Work out the finished part from the listing and answer in its coordinate system (mm). Face numbers are marked on the shaded views. Coordinates: 2 decimals unless noted, no trailing zeros. Order: outer loops, then holes, each group sorted by start corner. A loop starts at its lowest first (then second) coordinate and runs counter-clockwise, first axis right, second up. Notation, with made-up numbers: M -4,8.5 L 5,8.5 A15 cw 5,31.5 Z; hole C 23,85 d11. An arc over 180 degrees is marked long. Use a Markdown table: item, result.
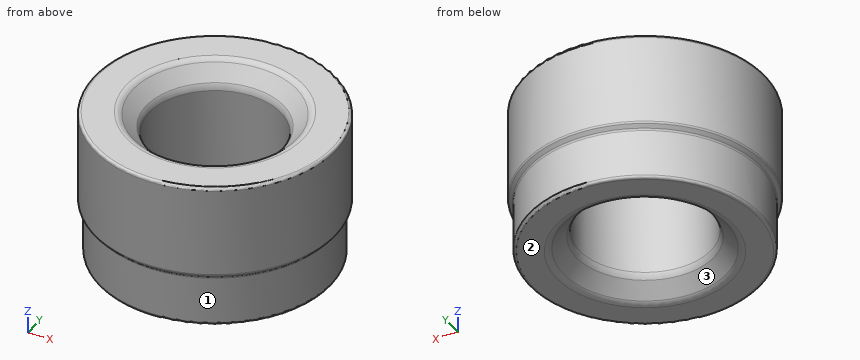
from build123d import *

# Parameters (mm, degrees)
SKETCH1_R           = 5
BOSS_EXTRUDE1_DEPTH = 2.76
SKETCH4_R           = 12.5
BOSS_EXTRUDE2_DEPTH = 6
SKETCH5_R           = 13
BOSS_EXTRUDE3_DEPTH = 10
FILLET2_R           = 0.3
FILLET3_R           = 0.3
SKETCH6_R           = 7.132829082
CUT_EXTRUDE1_DEPTH  = 31
CHAMFER1_SIZE       = 2
FILLET4_R           = 1
CHAMFER3_SIZE       = 0.5
FILLET7_R           = 0.3


with BuildPart() as part:
    # Sketch1 → Boss-Extrude1 (new body)
    with BuildSketch(Plane.XY):
        Circle(SKETCH1_R)
    extrude(amount=BOSS_EXTRUDE1_DEPTH)

    # Sketch4 → Boss-Extrude2 (add)
    with BuildSketch(Plane.XY.offset(2.76)):
        Circle(SKETCH4_R)
    extrude(amount=BOSS_EXTRUDE2_DEPTH)

    # Sketch5 → Boss-Extrude3 (add)
    with BuildSketch(Plane.XY.offset(8.76)):
        Circle(SKETCH5_R)
    extrude(amount=BOSS_EXTRUDE3_DEPTH)

    # Fillet2
    fillet2_edges = [part.edges().sort_by_distance(p)[0] for p in [
        (-5, 0, 2.76),
    ]]
    fillet(fillet2_edges, radius=FILLET2_R)

    # Fillet3
    fillet3_edges = [part.edges().sort_by_distance(p)[0] for p in [
        (-13, 0, 18.76),
    ]]
    fillet(fillet3_edges, radius=FILLET3_R)

    # Sketch6 → Cut-Extrude1 (cut)
    with BuildSketch(Plane.XY.offset(18.76)):
        Circle(SKETCH6_R)
    extrude(amount=-CUT_EXTRUDE1_DEPTH, mode=Mode.SUBTRACT)

    # Chamfer1
    chamfer1_edges = [part.edges().sort_by_distance(p)[0] for p in [
        (-7.132829082, 0, 2.76),
        (-7.132829082, 0, 18.76),
    ]]
    chamfer(chamfer1_edges, length=CHAMFER1_SIZE)

    # Fillet4
    fillet4_edges = [part.edges().sort_by_distance(p)[0] for p in [
        (-9.132829082, 0, 2.76),
        (-7.132829082, 0, 16.76),
        (-7.132829082, 0, 4.76),
        (-9.132829082, 0, 18.76),
    ]]
    fillet(fillet4_edges, radius=FILLET4_R)

    # Chamfer3
    chamfer3_edges = [part.edges().sort_by_distance(p)[0] for p in [
        (-12.5, 0, 8.76),
    ]]
    chamfer(chamfer3_edges, length=CHAMFER3_SIZE - 0.0001)  # a hair under: the kernel refuses the full size

    # Fillet6: read off the stored shape, not the designer's step
    # Fillet6 outline → Fillet6 (revolve, cut)
    with BuildSketch(Plane.XZ):
        with BuildLine():
            Line((13, 8.672132034), (13, 8.884264069))
            ThreePointArc((13, 8.884264069), (12.97716386, 8.769459039), (12.912132034, 8.672132034))
            Line((12.912132034, 8.672132034), (13, 8.672132034))
        make_face()
    revolve(axis=Axis((0, 0, 0), (0, 0, 1)), mode=Mode.SUBTRACT)

    # Fillet6 2 outline → Fillet6 2 (revolve)
    with BuildSketch(Plane.XZ):
        with BuildLine():
            ThreePointArc((12.5, 8.135735931), (12.52283614, 8.250540961), (12.587867966, 8.347867966))
            Line((12.587867966, 8.347867966), (12.5, 8.347867966))
            Line((12.5, 8.347867966), (12.5, 8.135735931))
        make_face()
    revolve(axis=Axis((0, 0, 0), (0, 0, 1)))

    # Fillet7
    fillet7_edges = [part.edges().sort_by_distance(p)[0] for p in [
        (-12.5, 0, 2.76),
    ]]
    fillet(fillet7_edges, radius=FILLET7_R)


solid = part.part
(1) Determine the mould class of the marked faces 1, 2 and 3 for opening direction X: pulls with the +X half, pulls with the -X half, needs draft (parallel to the pull), parting line crosses it, or undercut.
Conclusion:
| item | result |
|---|---|
| face 1 | parting line crosses it |
| face 2 | needs draft |
| face 3 | undercut |
(2) A cutting plane is placed at B-B (z = 10.5). Determine the outline of the cut face in (x, y), then the cut area to 3 significant figures.
Conclusion:
| item | result |
|---|---|
| outline | C 0,0 d26; hole C 0,0 d14.27 |
| area | 371 mm2 |
(3) Given P1, Ø3, axis at y = 3, z = 10, coming from the -X side; P2, Ø6, axis at x = -4.5, z = 5, coming from the +Y side; P3, Ø1.5, axis at x = -5, z = 5, coming from the +Y side, each flat-ended and moving along its own axis, determine where each tip first touches the part or whether it passes through.
Conclusion:
| item | result |
|---|---|
| P1 | x = -12.91 |
| P2 | y = 12.41 |
| P3 | y = 11.76 |
(4) Straight lines are drawn through the part: L1, parallel to Y at x = 0, z = 8; L2, parallel to Y at x = 0, z = 12.5; L3, parallel to X at y = -2, z = 5.75. For each, find the intervals that lie inside material, in ascending order.
Conclusion:
| item | result |
|---|---|
| L1 | -12.5 to -7.13, 7.13 to 12.5 |
| L2 | -13 to -7.13, 7.13 to 13 |
| L3 | -12.34 to -6.85, 6.85 to 12.34 |
(5) A cutting plane is placed at A-A (z = 5.75). Determine the outline of the cut face in (x, y).
Conclusion:
| item | result |
|---|---|
| outline | C 0,0 d25; hole C 0,0 d14.27 |
